Source: CAD feature listing. Evaluate the final solid. Frame: model axes, mm. Face numbers are marked on the shaded views. Round coordinates to 2 decimals unless told otherwise and drop trailing zeros. Loops run counter-clockwise (first coordinate to the right, second up) from the corner with the lowest first, then second, coordinate; pieces in that order, holes last.
(1) Section C-C, the plane z = -1.75. Return the cut outline in (x, y), plus the area to 3 significant figures.
(2) Section A-A, the plane y = -0.5. Count the separate pieces of the cut face and the enclosed holes in it, plus the area to 3 significant figures.
(3) Material intervals for probe 1 along X at (y, z) = (-9.25, 7.5); probe 2 along X at (y, z) = (-7, 6); probe 3 along Z at (x, y) = (17.5, -6), sorted ascending.
(4) Section B-B, the plane x = 6.35. Return the cut outline in (y, z) (3 decimals), plus the area to 3 significant figures.
(5) Mould query, pull axis Z, two halves, no side actions, for the marked faces 1, 2 and 3. Classes: pulls with the +Z half, pulls with the -Z half, needs draft (parallel to the pull), parting line crosses it, or undercut.
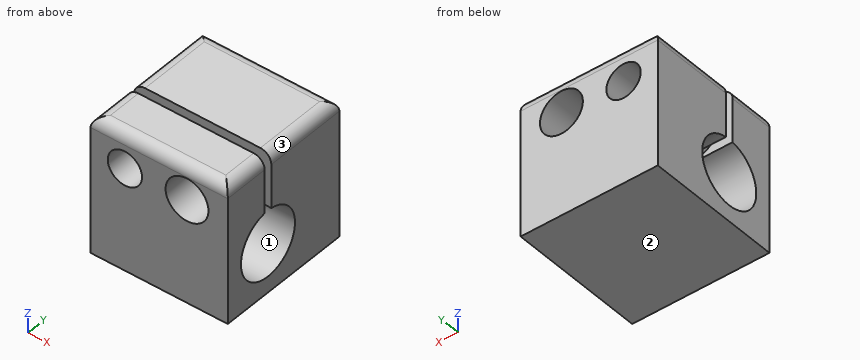
```python
from build123d import *

# Parameters (mm, degrees)
F1_DEPTH = 25.4
F2_R     = 3.175
F2_R_2   = 3.96875
F3_DEPTH = 25.401
F4_R     = 2.032


with BuildPart() as f1:
    # F0 (on Right) → F1 (new body)
    with BuildSketch(Plane.YZ):
        with BuildLine():
            Line((12.7, -12.7), (12.7, 12.7))
            Line((12.7, 12.7), (-2.794, 12.7))
            Line((-2.794, 12.7), (-2.794, 2.548185))
            ThreePointArc((-2.794, 2.548185), (-3.556, -9.707563), (-4.318, 2.548185))
            Line((-4.318, 2.548185), (-4.318, 12.7))
            Line((-4.318, 12.7), (-12.7, 12.7))
            Line((-12.7, 12.7), (-12.7, -12.7))
            Line((-12.7, -12.7), (12.7, -12.7))
        make_face()
    extrude(amount=F1_DEPTH)

    # F2 (on face) → F3 (cut, through all)
    with BuildSketch(Plane.XZ.offset(12.7)):
        with Locations((6.35, 6.35)):
            Circle(F2_R)
        with Locations((17.846059, 6.5024)):
            Circle(F2_R_2)
    extrude(amount=-F3_DEPTH, mode=Mode.SUBTRACT)

    # F4
    f4_edges = [f1.edges().sort_by_distance(p)[0] for p in [
        (0, 4.953, 12.7),
        (12.7, 12.7, 12.7),
        (25.4, 4.953, 12.7),
        (25.4, -8.509, 12.7),
        (12.7, -12.7, 12.7),
        (0, -8.509, 12.7),
    ]]
    fillet(f4_edges, radius=F4_R)


solid = f1.part
```
Output values:
1. outline: (0, -12.7) - (25.4, -12.7) - (25.4, -9.44) - (0, -9.44) - close; (0, 2.32) - (25.4, 2.32) - (25.4, 12.7) - (0, 12.7) - close
1. area: 346 mm2
2. separate pieces: 2
2. enclosed holes: 2
2. area: 291 mm2
3. probe 1: x = 0 to 3.39, 9.31 to 14, 21.69 to 25.4
3. probe 2: x = 0 to 3.19, 9.51 to 13.91, 21.78 to 25.4
3. probe 3: z = -12.7 to -9.2, 2.09 to 2.55, 10.46 to 12.7
4. outline: (-12.7, -12.7) - (12.7, -12.7) - (12.7, 3.175) - (-2.794, 3.175) - (-2.794, 2.548) arc R6.152 cw (long way) to (-4.318, 2.548) - (-4.318, 3.175) - (-12.7, 3.175) - close; (-12.7, 9.525) - (-4.318, 9.525) - (-4.318, 12.7) - (-10.668, 12.7) arc R2.032 ccw to (-12.7, 10.668) - close; (-2.794, 9.525) - (12.7, 9.525) - (12.7, 10.668) arc R2.032 ccw to (10.668, 12.7) - (-2.794, 12.7) - close
4. area: 357 mm2
5. face 1: undercut
5. face 2: pulls with the -Z half
5. face 3: pulls with the +Z half
